Here's how the part is built. I have some questions about the finished solid (model axes, mm). Face numbers are marked on the shaded views. A direction names the side the tool comes from. Round coordinates to 2 decimals unless told otherwise and drop trailing zeros. Order: outer loops, then holes, each group sorted by start corner. A loop starts at its lowest first (then second) coordinate and runs counter-clockwise, first axis right, second up.
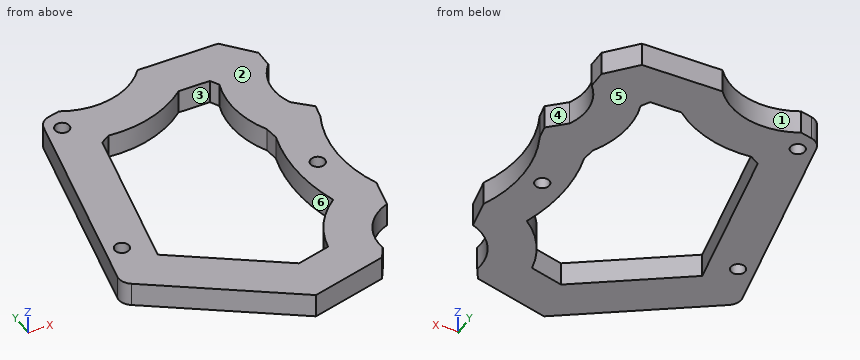
```python
from build123d import *

# Parameters (mm, degrees)
SKETCH2_R           = 1.5
BOSS_EXTRUDE1_DEPTH = 5
FILLET1_R           = 3
CHAMFER3_SIZE       = 2


with BuildPart() as part:
    # Sketch2 → Boss-Extrude1 (new body)
    with BuildSketch(Plane.XY.offset(-29.5)):
        with BuildLine():
            Line((-2.624619354, 3.548914368), (-11.801237054, -45.426295313))
            Line((-11.801237054, -45.426295313), (18.322008005, -65.275718381))
            Line((18.322008005, -65.275718381), (36.176514182, -60.587663687))
            ThreePointArc((36.176514182, -60.587663687), (36.583090059, -52.82338526), (42.360756545, -47.620703893))
            Line((42.360756545, -47.620703893), (43.567071105, -41.182655532))
            ThreePointArc((43.567071105, -41.182655532), (41.213039161, -30.088151018), (43.567071105, -18.993646503))
            Line((43.567071105, -18.993646503), (44.148406248, -16.06786198))
            Line((44.148406248, -16.06786198), (40.610484334, -12.837581299))
            ThreePointArc((40.610484334, -12.837581299), (39.645613087, -6.714468603), (42.210497415, -1.071344115))
            Line((42.210497415, -1.071344115), (42.210497415, 2.742539662))
            Line((42.210497415, 2.742539662), (36.882012848, 8.585085022))
            Line((36.882012848, 8.585085022), (20.167337536, 8.585085022))
            ThreePointArc((20.167337536, 8.585085022), (11.667192324, 3.260597998), (1.723711062, 4.575820826))
            Line((1.723711062, 4.575820826), (-2.624619354, 3.548914368))
        make_face()
        Circle(SKETCH2_R, mode=Mode.SUBTRACT)
        with Locations((36.882012848, -30.719979302)):
            Circle(SKETCH2_R, mode=Mode.SUBTRACT)
        with Locations((-6.752606997, -36.378596712)):
            Circle(SKETCH2_R, mode=Mode.SUBTRACT)
        with BuildLine():
            Line((-1.853309264, -41.203149553), (19.920649662, -55.5508907))
            Line((19.920649662, -55.5508907), (26.912648631, -53.715002702))
            ThreePointArc((26.912648631, -53.715002702), (29.448505151, -47.134631862), (34.193378933, -41.917542493))
            ThreePointArc((34.193378933, -41.917542493), (32.235117961, -31.354391616), (33.452553096, -20.680461028))
            Line((33.452553096, -20.680461028), (33.092400062, -17.875614172))
            ThreePointArc((33.092400062, -17.875614172), (30.652450166, -10.205517854), (31.469259091, -2.198236405))
            Line((31.469259091, -2.198236405), (30.430492401, -0.414914978))
            Line((30.430492401, -0.414914978), (23.934260151, -0.414914978))
            ThreePointArc((23.934260151, -0.414914978), (15.757383222, -4.951165755), (6.464186316, -5.988170424))
            Line((6.464186316, -5.988170424), (4.514445223, -7.21872072))
            Line((4.514445223, -7.21872072), (-1.853309264, -41.203149553))
        make_face(mode=Mode.SUBTRACT)
    extrude(amount=BOSS_EXTRUDE1_DEPTH)

    # Fillet1
    fillet1_edges = [part.edges().sort_by_distance(p)[0] for p in [
        (-11.801237054, -45.426295313, -27),
        (-2.624619354, 3.548914368, -27),
    ]]
    fillet(fillet1_edges, radius=FILLET1_R)

    # Chamfer3
    # the kernel refuses this chamfer: 2, 1.851821387 mm, written as the material it takes off along each edge
    with BuildSketch(Plane(origin=(36.176514182, -60.587663687, -34.731164248), x_dir=(-0.9672143762553561, -0.25396131667039873, 0), z_dir=(0, 0, 1))) as chamfer3_piece_1:
        with BuildLine():
            Line((CHAMFER3_SIZE, 0), (-0.03393884, -2.03393884))
            ThreePointArc((-0.03393884, -2.03393884), (0.03354605, -1.046793416), (0, 0))
            Line((0, 0), (CHAMFER3_SIZE, 0))
        make_face()
    extrude(amount=15.462328496, mode=Mode.SUBTRACT)


solid = part.part
```
1. If we section it at C-C, the plane y = -49: Write out the boundary of the cut face in (x, z), and give its area (3 significant figures).
Evaluation:
outline: (-6.38, -29.5) - (9.98, -29.5) - (9.98, -24.5) - (-6.38, -24.5) - close; (28.44, -29.5) - (39.75, -29.5) - (39.75, -24.5) - (28.44, -24.5) - close
area: 138 mm2
2. If we mould it in two halves opening along Y, with no side actions, what happens to the marked faces 1, 2 and 3? For each: released by +Y, released by -Y, zero draft, split by the parting line, or undercut.
Evaluation:
face 1: released by +Y
face 2: zero draft
face 3: undercut
3. If we section it at B-B, the plane z = -28: State how many separate pieces and enclosed holes the cut face has, and give its area (3 significant figures).
Evaluation:
separate pieces: 1
enclosed holes: 4
area: 1,690 mm2
4. I need wall thicknesses on probe 1 along X at (y, z) = (-35.5, -26.6); probe 2 along X at (y, z) = (-20.5, -25.6); probe 3 along Y at (x, z) = (13, -28.75). Which ranges of each line are inside material? Lowest first, please.
Evaluation:
probe 1: x = -9.94 to -7.97, -5.54 to -0.78, 32.62 to 41.75
probe 2: x = -7.13 to 2.03, 33.43 to 42.95
probe 3: y = -61.77 to -50.99, -5.65 to 3.62
5. I'm going to push flat-ended pins straight in: P1, Ø1.5, axis at x = 27.5, z = -26, coming from the -Y side; P2, Ø2.5, axis at x = 36.88, y = -30.72, coming from the -Z side; P3, Ø2, axis at x = 14, z = -28, coming from the +Y side (3 decimals); P4, Ø1.5, axis at x = 15, z = -28, coming from the -Y side. Where does each tip first touch, or does it pass through?
Evaluation:
P1: stops at y = -63.06
P2: passes through
P3: stops at y = 4.415
P4: stops at y = -63.58
6. On a 3-axis mill with a long thin cutter (end or side, diameter ignored), from which of +Z, -Z, +X, -X, +Y, -Y can I reach the whole of each face in a straight line? I mean the marked faces 4, 5 and 6. Say none if no direction works.
Evaluation:
face 4: +Z, -Z, +X
face 5: -Z, +X, -X, +Y, -Y
face 6: +Z, -Z
7. If we section it at A-A, the plane x = 15: Write out the boundary of the cut face in (y, z) (3 decimals), and give its area (3 significant figures).
Evaluation:
outline: (-63.087, -29.5) - (-52.308, -29.5) - (-52.308, -24.5) - (-63.087, -24.5) - close; (-5.179, -29.5) - (4.415, -29.5) - (4.415, -24.5) - (-5.179, -24.5) - close
area: 102 mm2
